The model under review builds one solid part; all positions refer to its coordinate system, in mm. Face numbers are marked on the shaded views. A direction names the side the tool comes from. Round coordinates to 2 decimals unless told otherwise and drop trailing zeros. Write each loop counter-clockwise with the first axis right and the second up, starting at its lowest first coordinate (ties: lowest second). Pieces come first, ordered by that corner, then holes.
Item 1: Add section C-C (x = 7.5). Give the boundary of the cut face in (y, z), plus the area to 3 significant figures.
Item 2: Machinability: for the marked faces 1 and 2, which of the approach directions +Z, -Z, +X, -X, +Y, -Y give a long, thin tool a straight path to every point of the face, cutting with its end or side? Answer none if there is none.
Item 3: Add section D-D (z = 15). Give the boundary of the cut face in (x, y).
Item 4: Add section B-B (z = 5). Give the boundary of the cut face in (x, y), plus the area to 3 significant figures.
Item 5: To check wall thickness, follow L1, parallel to Z at x = 7.5, y = -0.6; L2, parallel to X at y = -1.6, z = 5; L3, parallel to Y at x = 10.75, z = 8.5. State the ranges of each line that lie inside material, in increasing order.
Item 6: Clearance check with a flat-ended pin moving along its axis: pin 1 Ø6.5 at (y, z) = (-9, 15) entering from +X. State where the tip first meets the part, or that it passes through.
Item 7: Add section A-A (y = -9). Give the boundary of the cut face in (x, z).
```python
from build123d import *

# Parameters (mm, degrees)
EXTRUDE_1_DEPTH     = 30
SKETCH_2_R          = 1.6
CUT_EXTRUDE_1_DEPTH = 30
SKETCH_3_R          = 2.1
CUT_EXTRUDE_2_DEPTH = 30


with BuildPart() as part:
    # ｽｹｯﾁ1 → ﾎﾞｽ - 押し出し1 (new body)
    with BuildSketch(Plane.XY):
        Polygon((0, 0), (0, -15), (2, -15), (2, -2), (15, -2), (15, 0), align=None)
    extrude(amount=EXTRUDE_1_DEPTH)

    # ｽｹｯﾁ2 → ｶｯﾄ - 押し出し1 (cut)
    with BuildSketch(Plane(origin=(0, 0, 0), x_dir=(1, 0, 0), z_dir=(0, 1, 0))):
        with Locations((7.5, -5)):
            Circle(SKETCH_2_R)
        with Locations((7.5, -25)):
            Circle(SKETCH_2_R)
    extrude(amount=-CUT_EXTRUDE_1_DEPTH, mode=Mode.SUBTRACT)

    # ｽｹｯﾁ3 → ｶｯﾄ - 押し出し2 (cut)
    with BuildSketch(Plane.ZY):
        with Locations((15, -9)):
            Circle(SKETCH_3_R)
    extrude(amount=-CUT_EXTRUDE_2_DEPTH, mode=Mode.SUBTRACT)


solid = part.part
```
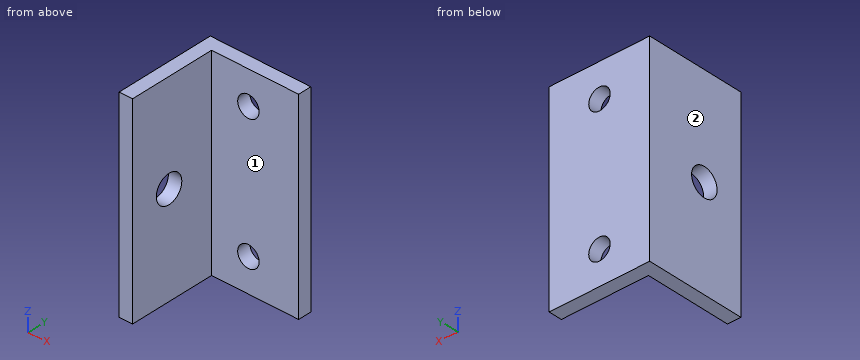
Numbers:
1. outline: (-2, 0) - (0, 0) - (0, 3.4) - (-2, 3.4) - close; (-2, 6.6) - (0, 6.6) - (0, 23.4) - (-2, 23.4) - close; (-2, 26.6) - (0, 26.6) - (0, 30) - (-2, 30) - close
1. area: 47.2 mm2
2. face 1: +Z, -Z, +X, -Y
2. face 2: +Z, -Z, -X, +Y, -Y
3. outline: (0, -15) - (2, -15) - (2, -11.1) - (0, -11.1) - close; (0, -6.9) - (2, -6.9) - (2, -2) - (15, -2) - (15, 0) - (0, 0) - close
4. outline: (0, -15) - (2, -15) - (2, -2) - (5.9, -2) - (5.9, 0) - (0, 0) - close; (9.1, -2) - (15, -2) - (15, 0) - (9.1, 0) - close
4. area: 49.6 mm2
5. L1: z = 0 to 3.4, 6.6 to 23.4, 26.6 to 30
5. L2: x = 0 to 5.9, 9.1 to 15
5. L3: y = -2 to 0
6. pin 1: stops at x = 2
7. outline: (0, 0) - (2, 0) - (2, 12.9) - (0, 12.9) - close; (0, 17.1) - (2, 17.1) - (2, 30) - (0, 30) - close
